from build123d import *

# Parameters (mm, degrees)
F0_R     = 6
F1_DEPTH = 75
F2_R     = 7
F2_R_2   = 6
F3_DEPTH = 1
F4_R     = 6
F5_DEPTH = 4
F7_D     = 6.8
F7_DEPTH = 15
F7_TIP   = 2.0429261047


with BuildPart() as f1:
    # F0 (on Front) → F1 (new body)
    with BuildSketch(Plane.XZ):
        Circle(F0_R)
    extrude(amount=F1_DEPTH)

    # F2 (on face) → F3 (join)
    with BuildSketch(Plane(origin=(0, 0, 0), x_dir=(-1, 0, 0), z_dir=(0, 1, 0))):
        Circle(F2_R)
        Circle(F2_R_2, mode=Mode.SUBTRACT)
        Circle(F2_R_2)
    extrude(amount=F3_DEPTH)

    # F4 (on face) → F5 (join)
    with BuildSketch(Plane(origin=(0, 1, 0), x_dir=(-1, 0, 0), z_dir=(0, 1, 0))):
        Circle(F4_R)
    extrude(amount=F5_DEPTH)

    # F7
    with Locations(Plane.XZ.offset(75)):
        with Locations((0, 0)):
            Hole(F7_D / 2, depth=F7_DEPTH)
            with Locations((0, 0, -(F7_DEPTH + F7_TIP / 2))):  # 118° drill point
                Cone(0, F7_D / 2, F7_TIP, mode=Mode.SUBTRACT)


solid = f1.part
Could you check a few things on this model? Use its own coordinates, in mm. A direction names the side the tool comes from. Give positions to 0.01 mm unless a question says otherwise; leave off trailing zeros. Order: outer loops, then holes, each group sorted by start corner. A loop starts at its lowest first (then second) coordinate and runs counter-clockwise, first axis right, second up. Notation, with made-up numbers: (-29, 6.25) - (20, 6.25) arc R33 ccw to (20, 45.25) - close; hole circle Ø4 at (-10, -36.5). An arc over 180 degrees is marked (long way). One line per item, written item: value. Start each with the question number.
1. For P1, Ø1, axis at x = -5, y = -53.5, coming from the -Z side; P2, Ø5, axis at x = -0.5, y = -59, coming from the +Z side; P3, Ø1.5, axis at x = -5.5, z = 3, coming from the +Y side; P4, Ø2, axis at y = -20, z = 1.5, coming from the +X side, each with a flat end and sliding along its axis, tell me the tip position at first contact or that it passes through.
2. Imagine slicing it at A-A on z = -5. List the corners of the cut face in (x, y) for me, plus the area to 3 significant figures.
3. Imagine slicing it at B-B on y = -30. List the corners of the cut face in (x, z) for me.
4. If I drill on probe 1 along Z at (x, y) = (0, -70); probe 2 along Y at (x, z) = (4.75, -4.75); probe 3 along X at (y, z) = (-67, 1.25), over which ranges is the centre line in solid material (lowest first)?
5. For faces 4 (the face through (0, 5, 0)), 5 (the face through (-6, 1, 2)), 6 (the face through (-6, 0, 2)), which set-ups out of +Z, -Z, +X, -X, +Y, -Y let a thin tool reach every point of the face, with its end or its side?
6. Thinking about a two-plate mould opening in X: for faces 1 (the face through (0.74, -67.4, -3.32)), 2 (the face through (3, -75, -3)), 3 (the face through (-6.466, 0.493, -2.681)), which applies, +X half, -X half, draft (parallel to the pull), parting line (faces both ways), or undercut?
Values:
1. P1: z = -3.97
1. P2: z = 6
1. P3: y = 5
1. P4: x = 5.98
2. outline: (-4.9, 0) - (-3.32, 0) - (-3.32, -75) - (3.32, -75) - (3.32, 0) - (4.9, 0) - (4.9, 1) - (3.32, 1) - (3.32, 5) - (-3.32, 5) - (-3.32, 1) - (-4.9, 1) - close
2. area: 534 mm²
3. outline: circle Ø12 at (0, 0)
4. probe 1: -6 to -3.4, 3.4 to 6
4. probe 2: 0 to 1
4. probe 3: -5.87 to -3.16, 3.16 to 5.87
5. face 4: +Z, -Z, +X, -X, +Y
5. face 5: +Y
5. face 6: -Y
6. face 1: undercut
6. face 2: draft
6. face 3: parting line
